Design review of the part built by this model. Coordinates are the model's own, in mm. A direction names the side the tool comes from. Round coordinates to 2 decimals unless told otherwise and drop trailing zeros. Order: outer loops, then holes, each group sorted by start corner. A loop starts at its lowest first (then second) coordinate and runs counter-clockwise, first axis right, second up. Notation, with made-up numbers: (49.25, 63) - (87.25, 63) arc R23 ccw to (87.25, 85) - close; hole circle Ø10 at (9, 83). An arc over 180 degrees is marked (long way). Use CSV: the item, a comma, the result in double quotes.
from build123d import *

# Parameters (mm, degrees)
F0_W     = 96.981816
F0_H     = 73.306844
F3_DEPTH = 25.4
F1_R     = 22.325888
F4_DEPTH = 63.5
F2_R     = 18.313732
F5_DEPTH = 63.501


with BuildPart() as f3:
    # F0 (on Front) → F3 (new body)
    with BuildSketch(Plane.XZ):
        Rectangle(F0_W, F0_H)
    extrude(amount=F3_DEPTH)

    # F1 (on face) → F4 (join)
    with BuildSketch(Plane.XZ):
        Circle(F1_R)
    extrude(amount=F4_DEPTH)

    # F2 (on face) → F5 (cut, through all)
    with BuildSketch(Plane.XZ):
        Circle(F2_R)
    extrude(amount=F5_DEPTH, mode=Mode.SUBTRACT)


solid = f3.part
1) For faces 4 (the face through (-22, -25.4, 9)), 5 (the face through (-48.491, -13, -1)), list the 3-axis set-ups (+Z, -Z, +X, -X, +Y, -Y) from which the entire face can be reached by the end or side of a thin tool; tool diameter is ignored.
Data:
face 4,"-Y"
face 5,"+Z, -Z, -X, +Y, -Y"
2) Insertion check: pin 1 Ø1.5 at (x, z) = (22.5, 21.5) entering from -Y; pin 2 Ø1.5 at (y, z) = (-41.5, 20.5) entering from +X; pin 3 Ø6 at (x, y) = (5.5, -56.5) entering from -Z. Each pin has a flat end and moves straight along its axis. Give the tip position at first contact, or say it passes through.
Data:
pin 1,"stops at y = -25.4"
pin 2,"stops at x = 10.41"
pin 3,"stops at z = -22.19"
3) We need section B-B (y = -21.5). Give the boundary of the cut face in (x, z), then the cut area to 3 significant figures.
Data:
outline,"(-48.49, -36.65) - (48.49, -36.65) - (48.49, 36.65) - (-48.49, 36.65) - close; hole circle Ø36.63 at (0, 0)"
area,"6,060 mm2"
4) We need section D-D (z = -31). Give the boundary of the cut face in (x, y), then the cut area to 3 significant figures.
Data:
outline,"(-48.49, -25.4) - (48.49, -25.4) - (48.49, 0) - (-48.49, 0) - close"
area,"2,460 mm2"
5) To check wall thickness, follow L1, parallel to Z at x = 0, y = -22; L2, parallel to X at y = -20.5, z = 0; L3, parallel to Z at x = 0, y = -44. State the ranges of each line that lie inside material, in increasing order. Write a range as from..to.
Data:
L1,"z = -36.65..-18.31, 18.31..36.65"
L2,"x = -48.49..-18.31, 18.31..48.49"
L3,"z = -22.33..-18.31, 18.31..22.33"
6) We need section A-A (z = 0). Give the boundary of the cut face in (x, y).
Data:
outline,"(-48.49, -25.4) - (-22.33, -25.4) - (-22.33, -63.5) - (-18.31, -63.5) - (-18.31, 0) - (-48.49, 0) - close; (18.31, -63.5) - (22.33, -63.5) - (22.33, -25.4) - (48.49, -25.4) - (48.49, 0) - (18.31, 0) - close"
7) The part is to be moulded in two halves that separate along Z. For faces 1 (the face through (-3.97, -31.31, -17.88)), 2 (the face through (-1, -13, 36.653)), 3 (the face through (-1, -13, -36.653)), say which applies: +Z half, -Z half, draft (parallel to the pull), parting line (faces both ways), or undercut.
Data:
face 1,"undercut"
face 2,"+Z half"
face 3,"-Z half"
8) We need section C-C (x = 0). Give the boundary of the cut face in (y, z).
Data:
outline,"(-63.5, -22.33) - (-25.4, -22.33) - (-25.4, -36.65) - (0, -36.65) - (0, -18.31) - (-63.5, -18.31) - close; (-63.5, 18.31) - (0, 18.31) - (0, 36.65) - (-25.4, 36.65) - (-25.4, 22.33) - (-63.5, 22.33) - close"
